Input: dimensioned drawing with shaded views. Units: mm. Origin: part minimum x, y, z. Round coordinates to 2 decimals unless told otherwise and drop trailing zeros. Write each loop counter-clockwise with the first axis right and the second up, starting at its lowest first coordinate (ties: lowest second). Pieces come first, ordered by that corner, then holes. Notation, with made-up numbers: (63.25, 1.25) -> (116.25, 1.25) arc R11 cw to (116.25, 7.25) -> close; hole circle Ø2 at (42.5, -25.5). An arc over 180 degrees is marked (long way). Use one line per item in the form item = value. Start each with the question number.
1. Pin query (flat end, axial travel): pin 1 Ø11 at (x, z) = (57.15, 19.05) entering from -Y; pin 2 Ø1 at (y, z) = (4, 29) entering from -X; pin 3 Ø1.5 at (y, z) = (3.5, 17.5) entering from -X. Return the tip coordinate at first contact, or that it passes through.
2. Cut plane D-D, the plane z = 19.05. Return the cut outline in (x, y), plus the area to 3 significant figures.
3. Cut plane A-A, the plane z = 95.25. Return the cut outline in (x, y), plus the area to 3 significant figures.
4. Cut plane B-B, the plane y = 1.75. State how many separate pieces and enclosed holes the cut face has, plus the area to 3 significant figures.
5. Line query: L1, parallel to X at y = 3, z = 95.25; L2, parallel to Z at x = 95.25, y = 2; L3, parallel to X at y = 1, z = 16. Output: solid intervals per line, ascending.
6. Cut plane C-C, the plane x = 133.35. Return the cut outline in (y, z).
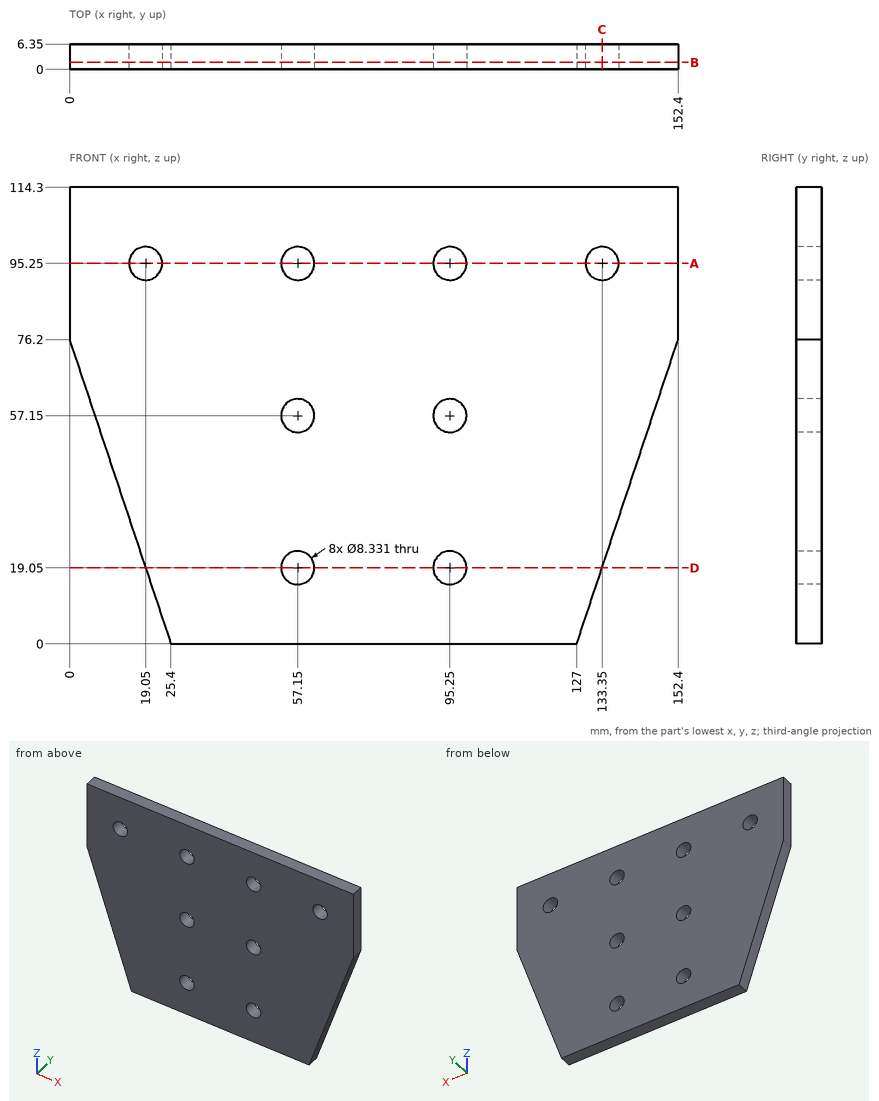
Outcome:
q1.pin_1 = 0
q1.pin_2 = 15.57
q1.pin_3 = 19.32
q2.outline = (19.05, 0) -> (52.98, 0) -> (52.98, 6.35) -> (19.05, 6.35) -> close; (61.32, 0) -> (91.08, 0) -> (91.08, 6.35) -> (61.32, 6.35) -> close; (99.42, 0) -> (133.35, 0) -> (133.35, 6.35) -> (99.42, 6.35) -> close
q2.area = 620 mm^2
q3.outline = (0, 0) -> (14.88, 0) -> (14.88, 6.35) -> (0, 6.35) -> close; (23.22, 0) -> (52.98, 0) -> (52.98, 6.35) -> (23.22, 6.35) -> close; (61.32, 0) -> (91.08, 0) -> (91.08, 6.35) -> (61.32, 6.35) -> close; (99.42, 0) -> (129.18, 0) -> (129.18, 6.35) -> (99.42, 6.35) -> close; (137.52, 0) -> (152.4, 0) -> (152.4, 6.35) -> (137.52, 6.35) -> close
q3.area = 756 mm^2
q4.separate_pieces = 1
q4.enclosed_holes = 8
q4.area = 15,000 mm^2
q5.L1 = 0 to 14.88, 23.22 to 52.98, 61.32 to 91.08, 99.42 to 129.18, 137.52 to 152.4
q5.L2 = 0 to 14.88, 23.22 to 52.98, 61.32 to 91.08, 99.42 to 114.3
q5.L3 = 20.07 to 54.31, 59.99 to 92.41, 98.09 to 132.33
q6.outline = (0, 19.05) -> (6.35, 19.05) -> (6.35, 91.08) -> (0, 91.08) -> close; (0, 99.42) -> (6.35, 99.42) -> (6.35, 114.3) -> (0, 114.3) -> close
